from build123d import *

# Parameters (mm, degrees)
SKETCH1_R                  = 11.1
BOSS_EXTRUDE1_DEPTH        = 3.8
BOSS_EXTRUDE2_START        = -3.8
SKETCH2_R                  = 5
BOSS_EXTRUDE2_DEPTH        = 14
SKETCH3_R                  = 4
CUT_EXTRUDE1_DEPTH         = 22.033782351
SKETCH4_R                  = 5.09
SKETCH4_R_2                = 4
BOSS_EXTRUDE3_DEPTH        = 1.67
F_3_5_3_5_DIAMETER_HOLE1_D = 3.5


with BuildPart() as part:
    # Sketch1 → Boss-Extrude1 (new body)
    with BuildSketch(Plane(origin=(0, 0, 0), x_dir=(1, 0, 0), z_dir=(0, 1, 0))):
        with Locations(Location((0, 0, 0), (0, 0, 90))):
            Circle(SKETCH1_R)
    extrude(amount=BOSS_EXTRUDE1_DEPTH)

    # Sketch2 → Boss-Extrude2 (add)
    with BuildSketch(Plane(origin=(0, 3.8, 0), x_dir=(1, 0, 0), z_dir=(0, 1, 0)).offset(BOSS_EXTRUDE2_START)):
        with Locations(Location((0, 0, 0), (0, 0, 270))):
            Circle(SKETCH2_R)
    extrude(amount=BOSS_EXTRUDE2_DEPTH)

    # Sketch3 → Cut-Extrude1 (cut, through all)
    with BuildSketch(Plane(origin=(0, 14, 0), x_dir=(1, 0, 0), z_dir=(0, 1, 0))):
        with Locations(Location((0, 0, 0), (0, 0, 270))):
            Circle(SKETCH3_R)
    extrude(amount=-CUT_EXTRUDE1_DEPTH, mode=Mode.SUBTRACT)

    # Sketch4 → Boss-Extrude3 (add)
    with BuildSketch(Plane.XZ):
        with Locations(Location((0, 0, 0), (0, 0, 90))):
            Circle(SKETCH4_R)
        with Locations(Location((0, 0, 0), (0, 0, 90))):
            Circle(SKETCH4_R_2, mode=Mode.SUBTRACT)
    extrude(amount=BOSS_EXTRUDE3_DEPTH)

    # Ø3.5 (3.5) Diameter Hole1 (through all)
    with Locations(Plane(origin=(0, 3.8, 0), x_dir=(1, 0, 0), z_dir=(0, 1, 0))):
        with Locations((0, 8), (0, -8), (8, 0), (-8, 0)):
            Hole(F_3_5_3_5_DIAMETER_HOLE1_D / 2)


solid = part.part
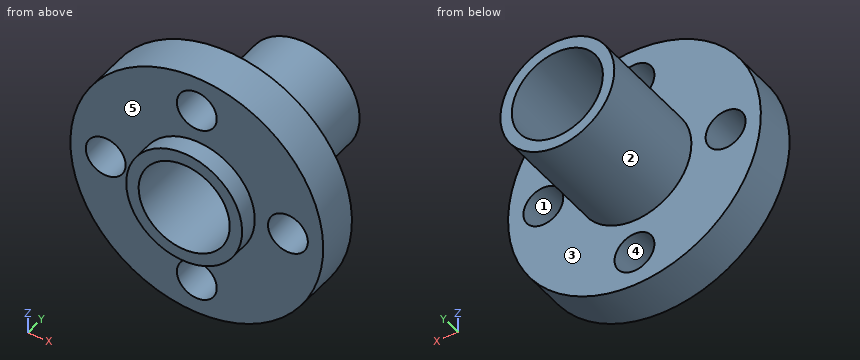
Could you check a few things on this model? Use its own coordinates, in mm. Face numbers are marked on the shaded views. A direction names the side the tool comes from. Give positions to 0.01 mm unless a question says otherwise; leave off trailing zeros. Loops run counter-clockwise (first coordinate to the right, second up) from the corner with the lowest first, then second, coordinate; pieces in that order, holes last. Notation, with made-up numbers: (-33.75, 11.25) -> (2.25, 11.25) arc R6 ccw to (2.25, 17.25) -> close; hole circle Ø2 at (86.5, 54). An arc over 180 degrees is marked (long way). Answer as CSV lines item,"result". Start each with the question number.
(1) I need wall thicknesses on probe 1 along Z at (x, y) = (0, 9); probe 2 along Y at (x, z) = (-8.5, -3.75); probe 3 along Z at (x, y) = (-8, 2.65). Which ranges of each line are inside material? Lowest first, please.
(2) We'd pull the mould along Z, two halves only. Please class the marked faces 1, 2 and 3: released by +Z, released by -Z, zero draft, split by the parting line, or undercut.
(3) If we section it at D-D on x = 8: Write out the boundary of the cut face in (y, z), then the cut area to 3 significant figures.
(4) Which directions (+Z, -Z, +X, -X, +Y, -Y) give clear straight access to the entire face, cutting with the end or side of a thin tool? Please do the marked faces 4 and 5.
(5) If we section it at A-A on x = 0: Write out the boundary of the cut face in (y, z).
(6) If we section it at B-B on z = 0: Write out the boundary of the cut face in (x, y).
(7) If we section it at C-C on y = 0.5: Write out the boundary of the cut face in (x, z).
(8) I'm going to push flat-ended pins straight in: pin 1 Ø1 at (x, y) = (0.5, 10.5) entering from -Z; pin 2 Ø3 at (y, z) = (5.5, 5) entering from -X; pin 3 Ø3 at (x, z) = (-8, 0) entering from -Y; pin 4 Ø8 at (x, y) = (1, 1.5) entering from +Z. Where does each tip first touch, or does it pass through?
Computed:
1,probe 1,"z = -5 to -4, 4 to 5"
1,probe 2,"y = 0 to 3.8"
1,probe 3,"z = -7.69 to -1.75, 1.75 to 7.69"
2,face 1,"undercut"
2,face 2,"split by the parting line"
2,face 3,"zero draft"
3,outline,"(0, -7.69) -> (3.8, -7.69) -> (3.8, -1.75) -> (0, -1.75) -> close; (0, 1.75) -> (3.8, 1.75) -> (3.8, 7.69) -> (0, 7.69) -> close"
3,area,"45.2 mm2"
4,face 4,"+Y, -Y"
4,face 5,"-Y"
5,outline,"(-1.67, -5.09) -> (0, -5.09) -> (0, -6.25) -> (3.8, -6.25) -> (3.8, -5) -> (14, -5) -> (14, -4) -> (-1.67, -4) -> close; (-1.67, 4) -> (14, 4) -> (14, 5) -> (3.8, 5) -> (3.8, 6.25) -> (0, 6.25) -> (0, 5.09) -> (-1.67, 5.09) -> close; (0, -11.1) -> (3.8, -11.1) -> (3.8, -9.75) -> (0, -9.75) -> close; (0, 9.75) -> (3.8, 9.75) -> (3.8, 11.1) -> (0, 11.1) -> close"
6,outline,"(-11.1, 0) -> (-9.75, 0) -> (-9.75, 3.8) -> (-11.1, 3.8) -> close; (-6.25, 0) -> (-5.09, 0) -> (-5.09, -1.67) -> (-4, -1.67) -> (-4, 14) -> (-5, 14) -> (-5, 3.8) -> (-6.25, 3.8) -> close; (4, -1.67) -> (5.09, -1.67) -> (5.09, 0) -> (6.25, 0) -> (6.25, 3.8) -> (5, 3.8) -> (5, 14) -> (4, 14) -> close; (9.75, 0) -> (11.1, 0) -> (11.1, 3.8) -> (9.75, 3.8) -> close"
7,outline,"circle Ø22.2 at (0, 0); hole circle Ø3.5 at (-8, 0); hole circle Ø8 at (0, 0); hole circle Ø3.5 at (0, -8); hole circle Ø3.5 at (0, 8); hole circle Ø3.5 at (8, 0)"
8,pin 1,"stops at z = -5"
8,pin 2,"stops at x = -3.57"
8,pin 3,"passes through"
8,pin 4,"stops at z = 11.1"
